```python
from build123d import *

# Parameters (mm, degrees)
F0_W     = 108.40325
F0_H     = 119.467252
F1_DEPTH = 25.4
F2_R     = 17.467659
F3_DEPTH = 25.4
F5_DEPTH = 119.468251


with BuildPart() as f1:
    # F0 (on Top) → F1 (new body)
    with BuildSketch(Plane.XY):
        Rectangle(F0_W, F0_H)
    extrude(amount=F1_DEPTH)

    # F2 (on face) → F3 (join)
    with BuildSketch(Plane.XY.offset(25.4)):
        Circle(F2_R)
    extrude(amount=F3_DEPTH)

    # F4 (on face) → F5 (cut, through all)
    with BuildSketch(Plane.XZ.offset(59.733626)):
        Polygon((17.467659, 50.8), (-17.467659, 50.8), (17.467659, 31.459402), align=None)
    extrude(amount=-F5_DEPTH, mode=Mode.SUBTRACT)


solid = f1.part
```
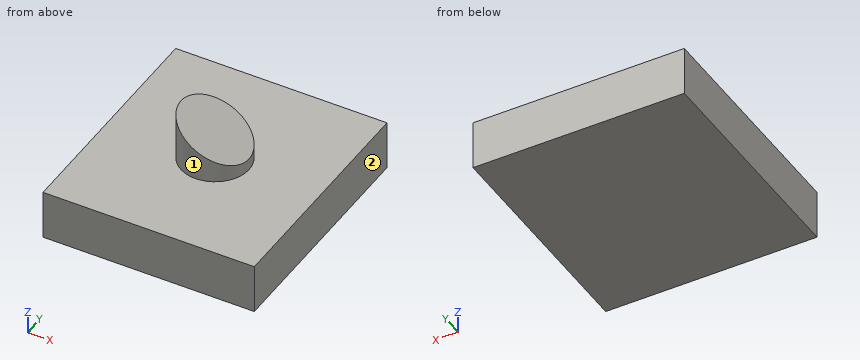
Can you work these out from the model? Positions are in its coordinate system, mm. Face numbers are marked on the shaded views. A direction names the side the tool comes from. Give positions to 0.01 mm unless a question says otherwise; leave off trailing zeros. Order: outer loops, then holes, each group sorted by start corner. A loop starts at its lowest first (then second) coordinate and runs counter-clockwise, first axis right, second up. Notation, with made-up numbers: M 28,-24.75 L 74,-24.75 A30 cw 74,9.25 Z; hole C 57,43.5 d4. An arc over 180 degrees is marked long. Write item = value, one per line. Start each with the question number.
Q1. Suppose I cut it at A-A (y = 0). Write out the boundary of the cut face in (x, z), plus the area to 3 significant figures.
Q2. I need wall thicknesses on probe 1 along Z at (x, y) = (38, -44.5); probe 2 along X at (y, z) = (-12, 38); probe 3 along Z at (x, y) = (12, 5.5). Which ranges of each line are inside material? Lowest first, please. Write a range as [from, to].
Q3. Suppose I cut it at C-C (x = 8). Write out the boundary of the cut face in (y, z).
Q4. Suppose I cut it at D-D (y = -40). Write out the boundary of the cut face in (x, z), plus the area to 3 significant figures.
Q5. Will this pin go through, and if not, where does the flat tip stop? pin 1 Ø4 at (x, y) = (11.5, 32) entering from +Z.
Q6. Suppose I cut it at B-B (z = 27.5). Write out the boundary of the cut face in (x, y), plus the area to 3 significant figures.
Q7. For the marked faces 1 and 2, which set-ups out of +Z, -Z, +X, -X, +Y, -Y let a thin tool reach every point of the face, with its end or its side?
Check result:
q1.outline = M -54.2,0 L 54.2,0 L 54.2,25.4 L 17.47,25.4 L 17.47,31.46 L -17.47,50.8 L -17.47,25.4 L -54.2,25.4 Z
q1.area = 3,300 mm2
q2.probe_1 = [0, 25.4]
q2.probe_2 = [-12.69, 5.65]
q2.probe_3 = [0, 34.49]
q3.outline = M -59.73,0 L 59.73,0 L 59.73,25.4 L 15.53,25.4 L 15.53,36.7 L -15.53,36.7 L -15.53,25.4 L -59.73,25.4 Z
q4.outline = M -54.2,0 L 54.2,0 L 54.2,25.4 L -54.2,25.4 Z
q4.area = 2,750 mm2
q5.pin_1 = 25.4
q6.outline = C 0,0 d34.94
q6.area = 959 mm2
q7.face_1 = +Z
q7.face_2 = +Z, -Z, +X, +Y, -Y
